```python
from build123d import *

# Parameters (mm, degrees)
SKETCH1_W           = 100
SKETCH1_H           = 80
SKETCH1_W_2         = 92.5
SKETCH1_H_2         = 74
BOSS_EXTRUDE1_DEPTH = 60
SKETCH2_W           = 92.5
SKETCH2_H           = 3
BOSS_EXTRUDE2_DEPTH = 77
SKETCH3_W           = 92.5
SKETCH3_H           = 3
BOSS_EXTRUDE3_DEPTH = 77
SKETCH4_W           = 54
SKETCH4_H           = 74
CUT_EXTRUDE1_DEPTH  = 77
SKETCH7_R           = 7.5
CUT_EXTRUDE2_DEPTH  = 10


with BuildPart() as part:
    # Sketch1 → Boss-Extrude1 (new body)
    with BuildSketch(Plane.XY):
        Rectangle(SKETCH1_W, SKETCH1_H)
        Rectangle(SKETCH1_W_2, SKETCH1_H_2, mode=Mode.SUBTRACT)
    extrude(amount=BOSS_EXTRUDE1_DEPTH)

    # Sketch2 → Boss-Extrude2 (add)
    with BuildSketch(Plane(origin=(0, -37, 0), x_dir=(1, 0, 0), z_dir=(0, 1, 0))):
        with Locations((0, -1.5)):
            Rectangle(SKETCH2_W, SKETCH2_H)
    extrude(amount=BOSS_EXTRUDE2_DEPTH)

    # Sketch3 → Boss-Extrude3 (add)
    with BuildSketch(Plane(origin=(0, -37, 0), x_dir=(1, 0, 0), z_dir=(0, 1, 0))):
        with Locations((0, -58.5)):
            Rectangle(SKETCH3_W, SKETCH3_H)
    extrude(amount=BOSS_EXTRUDE3_DEPTH)

    # Sketch4 → Cut-Extrude1 (cut)
    with BuildSketch(Plane(origin=(50, 0, 0), x_dir=(0, 0, -1), z_dir=(1, 0, 0))):
        with Locations((-30, 0)):
            Rectangle(SKETCH4_W, SKETCH4_H)
    extrude(amount=-CUT_EXTRUDE1_DEPTH, mode=Mode.SUBTRACT)

    # Sketch7 → Cut-Extrude2 (cut)
    with BuildSketch(Plane.XY.offset(60)):
        with BuildLine():
            ThreePointArc((11, 0), (18.5, -7.5), (26, 0))
            Line((26, 0), (18.5, 0))
            Line((18.5, 0), (11, 0))
        make_face()
        with BuildLine():
            Line((18.5, 0), (26, 0))
            ThreePointArc((26, 0), (18.5, 7.5), (11, 0))
            Line((11, 0), (18.5, 0))
        make_face()
        with Locations((-18.5, 0)):
            Circle(SKETCH7_R)
    extrude(amount=-CUT_EXTRUDE2_DEPTH, mode=Mode.SUBTRACT)


solid = part.part
```
Read the model definition and answer for the solid it produces. Units are mm, in the model's axes. A direction names the side the tool comes from. Coordinates: 2 decimals unless noted, no trailing zeros. Order: outer loops, then holes, each group sorted by start corner. A loop starts at its lowest first (then second) coordinate and runs counter-clockwise, first axis right, second up. Notation, with made-up numbers: (-24.75, -38) - (2.25, -38) arc R24 cw to (2.25, -8) - close; hole circle Ø9 at (75.25, 47.5). An arc over 180 degrees is marked (long way). Answer as a JSON object with one key per item and string values. Group by question number.
Item 1: Section B-B (x = 1.5) is taken. Give the vertices of the cut face in (y, z).
Item 2: Section A-A (z = 16.5) is taken. Give the vertices of the cut face in (x, y), plus the area to 4 significant figures.
Item 3: Section C-C (y = -4) is taken. Give the vertices of the cut face in (x, z).
Item 4: Flat-ended cylindrical pins translate along their axes: P1, Ø6, axis at x = 9.5, y = -4, coming from the -Z side; P2, Ø5, axis at y = -16, z = 7.5, coming from the +X side. Find the tip coordinate at first contact, or state that the pin passes through.
Item 5: Consider probe 1 along Y at (x, z) = (-26.5, 45); probe 2 along Z at (x, y) = (-27.5, -31.5); probe 3 along Y at (x, z) = (-18.5, 58.55). Determine where each line is inside the solid, lowest interval first. Write a range as from..to.
Item 6: Section D-D (x = -18.5) is taken. Give the vertices of the cut face in (y, z).
Item 7: A tool of negligible diameter and unlimited length cuts with its end or side. For faces 1 (the face through (-50, -1, 30)), 2 (the face through (-26, 0, 59)), 3 (the face through (3, -37, 30)), from which of +Z, -Z, +X, -X, +Y, -Y can it reach the whole face along a straight path? Write none if from no direction.
Item 8: The mould has two halves that part along Z. Classify faces 4 (the face through (3, -1, 57)), 5 (the face through (-1, -1, 60)), 6 (the face through (50, -3, 59)): +Z half, -Z half, draft (parallel to the pull), parting line (faces both ways), or undercut.
Results are:
{
 "1": {"outline": "(-40, 0) - (40, 0) - (40, 60) - (-40, 60) - close; hole (-37, 3) - (37, 3) - (37, 57) - (-37, 57) - close"},
 "2": {"outline": "(-50, -40) - (50, -40) - (50, -37) - (-46.25, -37) - (-46.25, 37) - (50, 37) - (50, 40) - (-50, 40) - close", "area": "877.5 mm^2"},
 "3": {"outline": "(-50, 0) - (50, 0) - (50, 3) - (-46.25, 3) - (-46.25, 57) - (-24.84, 57) - (-24.84, 60) - (-50, 60) - close; (-12.16, 57) - (12.16, 57) - (12.16, 60) - (-12.16, 60) - close; (24.84, 57) - (50, 57) - (50, 60) - (24.84, 60) - close"},
 "4": {"P1": "stops at z = 0", "P2": "stops at x = -46.25"},
 "5": {"probe 1": "y = -40..-37, 37..40", "probe 2": "z = 0..3, 57..60", "probe 3": "y = -40..-7.5, 7.5..40"},
 "6": {"outline": "(-40, 0) - (40, 0) - (40, 60) - (7.5, 60) - (7.5, 57) - (37, 57) - (37, 3) - (-37, 3) - (-37, 57) - (-7.5, 57) - (-7.5, 60) - (-40, 60) - close"},
 "7": {"face 1": "+Z, -Z, -X, +Y, -Y", "face 2": "+Z", "face 3": "+X"},
 "8": {"face 4": "undercut", "face 5": "+Z half", "face 6": "draft"}
}
